Answer from the drawing. Dimensions are ordinates in mm from the lowest x, y and z of the part. Coordinates: 2 decimals unless noted, no trailing zeros. Write each loop counter-clockwise with the first axis right and the second up, starting at its lowest first coordinate (ties: lowest second). Pieces come first, ordered by that corner, then holes.
1) Determine the mould class of the marked faces 1, 2 and 3 for opening direction Z: +Z half, -Z half, draft (parallel to the pull), parting line (faces both ways), or undercut.
2) Each of these flat-tipped pins is pushed along its axis until it touches: pin 1 Ø8 at (y, z) = (24, 29.5) entering from -X; pin 2 Ø5 at (x, z) = (9, 95) entering from -Y; pin 3 Ø3 at (x, y) = (8.5, 18.5) entering from -Z; pin 4 Ø10 at (x, z) = (11, 44) entering from +Y. Where does it stop, or does it pass through?
3) The part is cut by section D-D (x = 10.5). Determine the outline of the cut face in (y, z) (1 decimal).
4) Find the intervals of material crossed by line 1 (Z direction, x = 13, y = 10) (1 decimal); line 2 (Z direction, x = 31.5, y = 4) (1 decimal); line 3 (X direction, y = 41, z = 29) (1 decimal), in increasing order.
5) The part is cut by section C-C (z = 105). Determine the outline of the cut face in (x, y) (1 decimal), then the cut area to 4 significant figures.
6) The part is cut by section B-B (y = 25.4). Determine the outline of the cut face in (x, z) (1 decimal), then the cut area to 3 significant figures.
7) The part is cut by section A-A (x = 25.4). Determine the outline of the cut face in (y, z) (1 decimal).
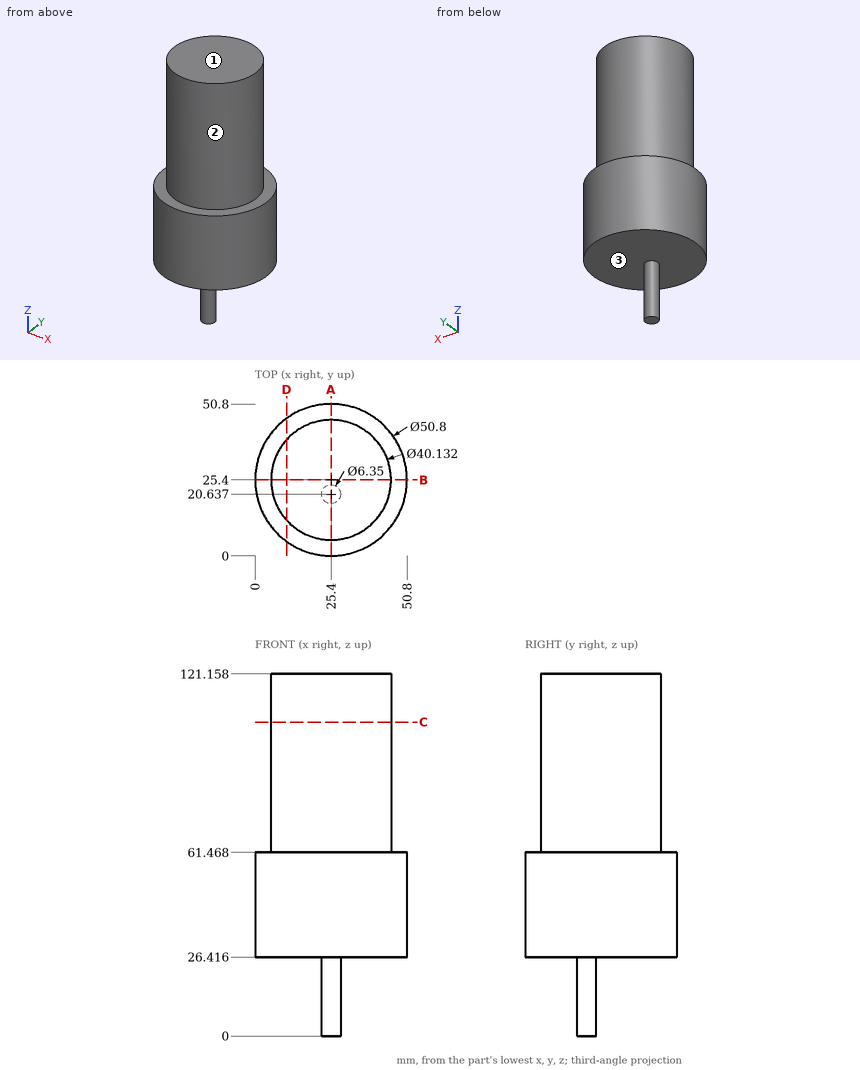
Reported:
1. face 1: +Z half
1. face 2: draft
1. face 3: -Z half
2. pin 1: stops at x = 0
2. pin 2: stops at y = 10.93
2. pin 3: stops at z = 26.42
2. pin 4: stops at y = 49
3. outline: (4.8, 26.4) - (46, 26.4) - (46, 61.5) - (38.8, 61.5) - (38.8, 121.2) - (12, 121.2) - (12, 61.5) - (4.8, 61.5) - close
4. line 1: z = 26.4 to 121.2
4. line 2: z = 26.4 to 61.5
4. line 3: x = 5.4 to 45.4
5. outline: circle Ø40.1 at (25.4, 25.4)
5. area: 1,265 mm2
6. outline: (0, 26.4) - (50.8, 26.4) - (50.8, 61.5) - (45.5, 61.5) - (45.5, 121.2) - (5.3, 121.2) - (5.3, 61.5) - (0, 61.5) - close
6. area: 4,180 mm2
7. outline: (0, 26.4) - (17.5, 26.4) - (17.5, 0) - (23.8, 0) - (23.8, 26.4) - (50.8, 26.4) - (50.8, 61.5) - (45.5, 61.5) - (45.5, 121.2) - (5.3, 121.2) - (5.3, 61.5) - (0, 61.5) - close
